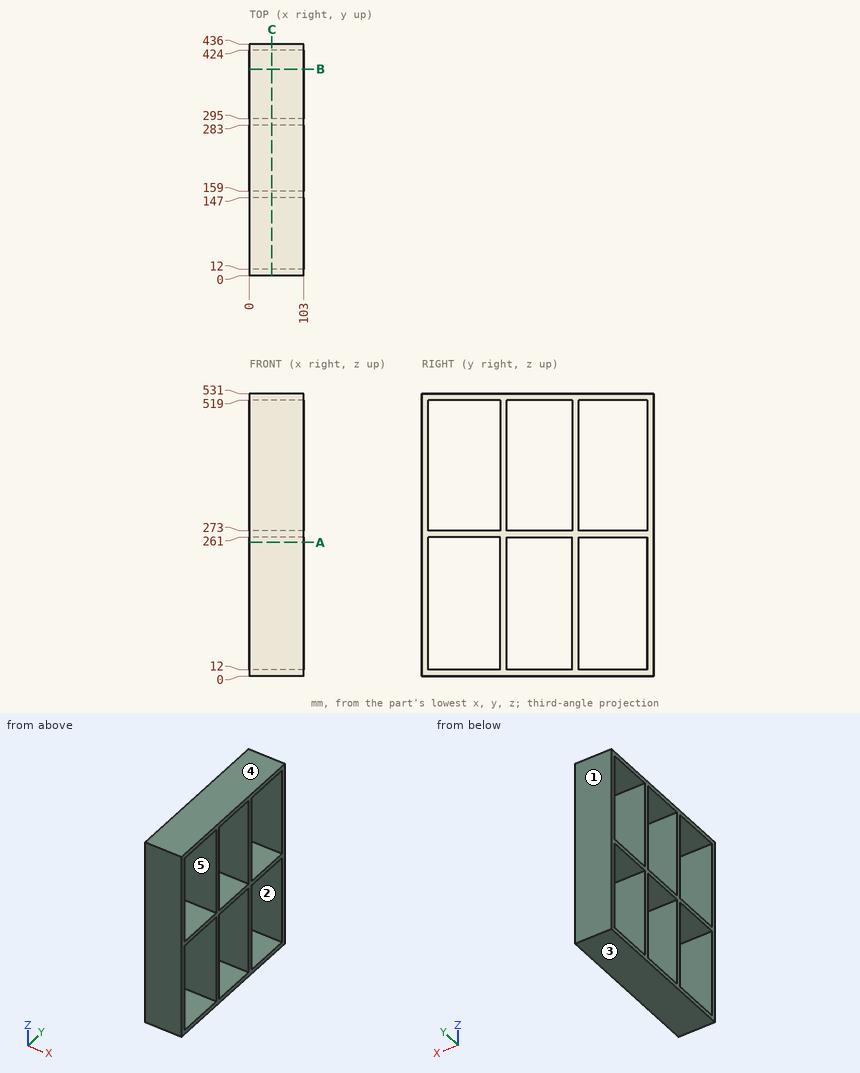
Design review of the part shown in the three views and the two pictorial views. Dimensions are in mm from the part's minimum x, y and z. A direction names the side the tool comes from. Give positions to 0.01 mm unless a question says otherwise; leave off trailing zeros. Loops run counter-clockwise (first coordinate to the right, second up) from the corner with the lowest first, then second, coordinate; pieces in that order, holes last. Notation, with made-up numbers: (34.5, -35.5) -> (48.5, -35.5) arc R33 ccw to (48.5, -2.5) -> close; hole circle Ø1 at (-28.75, 48). An arc over 180 degrees is marked (long way). Answer as a JSON object with one key per item and string values. Group by question number.
Q1. Take a section at B-B (y = 388.5). Write out the cut boundary in (x, z), plus the area to 3 significant figures.
Q2. Wall thickness on line 1 along Y through (x, z) = (37.5, 281); line 2 along Z through (x, y) = (33, 170): over which ranges is each line inside the solid? List them lowest first.
Q3. Take a section at C-C (x = 42.5). Write out the cut boundary in (y, z).
Q4. Insertion check: pin 1 (2 mm diameter, centred on x = 31.5, z = 90, fed in from -Y). The pin has a flat end and moves straight along its axis. Give the tip position at first contact, or say it passes through.
Q5. Tool access review of the marked faces 4 and 5: name each direction out of +Z, -Z, +X, -X, +Y, -Y from which nothing blocks a thin tool from reaching the whole face with its end or side.
Q6. Draft analysis for pull direction Y (two halves, no side actions). For the marked faces 1, 2 and 3, state which applies: pulls with the +Y half, pulls with the -Y half, needs draft (parallel to the pull), parting line crosses it, or undercut.
Q7. Take a section at A-A (z = 251.5). Write out the cut boundary in (x, y), plus the area to 3 significant figures.
Answer below:
{
 "1": {"outline": "(0, 0) -> (103, 0) -> (103, 12) -> (0, 12) -> close; (0, 261) -> (103, 261) -> (103, 273) -> (0, 273) -> close; (0, 519) -> (103, 519) -> (103, 531) -> (0, 531) -> close", "area": "3,710 mm2"},
 "2": {"line 1": "y = 0 to 12, 147 to 159, 283 to 295, 424 to 436", "line 2": "z = 0 to 12, 261 to 273, 519 to 531"},
 "3": {"outline": "(0, 0) -> (436, 0) -> (436, 531) -> (0, 531) -> close; hole (12, 12) -> (147, 12) -> (147, 261) -> (12, 261) -> close; hole (12, 273) -> (147, 273) -> (147, 519) -> (12, 519) -> close; hole (159, 12) -> (283, 12) -> (283, 261) -> (159, 261) -> close; hole (159, 273) -> (283, 273) -> (283, 519) -> (159, 519) -> close; hole (295, 12) -> (424, 12) -> (424, 261) -> (295, 261) -> close; hole (295, 273) -> (424, 273) -> (424, 519) -> (295, 519) -> close"},
 "4": {"pin 1": "stops at y = 0"},
 "5": {"face 4": "+Z, +X, -X, +Y, -Y", "face 5": "+X, -X"},
 "6": {"face 1": "pulls with the +Y half", "face 2": "undercut", "face 3": "needs draft"},
 "7": {"outline": "(0, 0) -> (103, 0) -> (103, 12) -> (0, 12) -> close; (0, 147) -> (103, 147) -> (103, 159) -> (0, 159) -> close; (0, 283) -> (103, 283) -> (103, 295) -> (0, 295) -> close; (0, 424) -> (103, 424) -> (103, 436) -> (0, 436) -> close", "area": "4,940 mm2"}
}
